from build123d import *

# Parameters (mm, degrees)
CROQUIS1_W              = 65
CROQUIS1_H              = 150
CROQUIS1_R              = 1.8
SALIENTE_EXTRUIR1_DEPTH = 2
CROQUIS2_W              = 3
CROQUIS2_H              = 150
SALIENTE_EXTRUIR2_DEPTH = 45
CROQUIS3_R              = 5.3
CROQUIS3_R_2            = 1.8
CORTAR_EXTRUIR1_DEPTH   = 10


with BuildPart() as part:
    # Croquis1 → Saliente-Extruir1 (new body)
    with BuildSketch(Plane(origin=(0, 0, 0), x_dir=(1, 0, 0), z_dir=(0, 1, 0))):
        Rectangle(CROQUIS1_W, CROQUIS1_H)
        with Locations(Location((-2.7, 12.25, 0), (0, 0, 270))):
            Circle(CROQUIS1_R, mode=Mode.SUBTRACT)
        with Locations(Location((-2.7, 60.57, 0), (0, 0, 270))):
            Circle(CROQUIS1_R, mode=Mode.SUBTRACT)
        with Locations(Location((-12.7, -60.57, 0), (0, 0, 90))):
            Circle(CROQUIS1_R, mode=Mode.SUBTRACT)
        with Locations(Location((-2.7, -60.57, 0), (0, 0, 90))):
            Circle(CROQUIS1_R, mode=Mode.SUBTRACT)
        with Locations(Location((-12.7, 12.25, 0), (0, 0, 270))):
            Circle(CROQUIS1_R, mode=Mode.SUBTRACT)
        with Locations(Location((-12.7, 60.57, 0), (0, 0, 270))):
            Circle(CROQUIS1_R, mode=Mode.SUBTRACT)
        with Locations(Location((-12.7, -12.25, 0), (0, 0, 90))):
            Circle(CROQUIS1_R, mode=Mode.SUBTRACT)
        with Locations(Location((-2.7, -12.25, 0), (0, 0, 90))):
            Circle(CROQUIS1_R, mode=Mode.SUBTRACT)
    extrude(amount=SALIENTE_EXTRUIR1_DEPTH)

    # Croquis2 → Saliente-Extruir2 (add)
    with BuildSketch(Plane(origin=(0, 2, 0), x_dir=(1, 0, 0), z_dir=(0, 1, 0))):
        with Locations((31, 0)):
            Rectangle(CROQUIS2_W, CROQUIS2_H)
    extrude(amount=SALIENTE_EXTRUIR2_DEPTH)

    # Croquis3 → Cortar-Extruir1 (cut)
    with BuildSketch(Plane(origin=(32.5, 0, 0), x_dir=(0, 0, -1), z_dir=(1, 0, 0))):
        with Locations((0, 23.5)):
            Circle(CROQUIS3_R)
        with Locations((-7.424621202, 16.075378798)):
            Circle(CROQUIS3_R_2)
        with Locations((-7.424621202, 30.924621202)):
            Circle(CROQUIS3_R_2)
        with Locations((7.424621202, 30.924621202)):
            Circle(CROQUIS3_R_2)
        with Locations((7.424621202, 16.075378798)):
            Circle(CROQUIS3_R_2)
    extrude(amount=-CORTAR_EXTRUIR1_DEPTH, mode=Mode.SUBTRACT)


solid = part.part
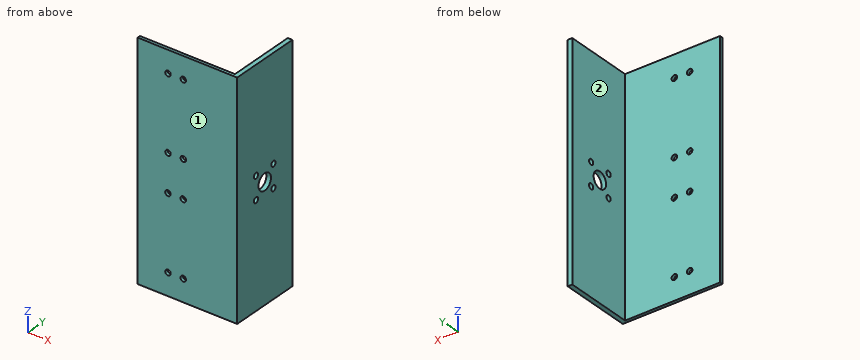
Build history of the part. All positions in model axes, mm. Face numbers are marked on the shaded views. A direction names the side the tool comes from. Coordinates: 2 decimals unless noted, no trailing zeros. Write each loop counter-clockwise with the first axis right and the second up, starting at its lowest first coordinate (ties: lowest second). Pieces come first, ordered by that corner, then holes.
(1) Pin check, flat tips, straight feed: pin 1 Ø17 at (y, z) = (23.5, 0) entering from +X; pin 2 Ø1 at (x, z) = (-18.5, 38.5) entering from +Y; pin 3 Ø8 at (y, z) = (36, -37) entering from -X. Stop position of each tip, or through.
(2) Cut at D-D on z = 41.5. List the corners of the cut face in (x, y), and give its area (3 significant figures).
(3) Cut at A-A on z = 0. List the corners of the cut face in (x, y), and give its area (3 significant figures).
(4) Cut at C-C on y = 23.5. List the corners of the cut face in (x, z).
(5) Drill centre lines: line 1 (X direction, y = 1, z = 12); line 2 (Y direction, x = 31.55, z = 0); line 3 (Y direction, x = 2, z = -32). Where is each one in solid material? Low to high.
(6) Cut at B-B on x = -2.7. List the corners of the cut face in (y, z).
(7) 3-axis set-ups, long thin cutter, end or side, ignore diameter. For the marked faces 1 and 2: which of +Z, -Z, +X, -X, +Y, -Y reach the whole face in a straight line?
Working result:
1. pin 1: stops at x = 32.5
1. pin 2: stops at y = 2
1. pin 3: stops at x = 29.5
2. outline: (-32.5, 0) - (32.5, 0) - (32.5, 47) - (29.5, 47) - (29.5, 2) - (-32.5, 2) - close
2. area: 265 mm2
3. outline: (-32.5, 0) - (32.5, 0) - (32.5, 18.2) - (29.5, 18.2) - (29.5, 2) - (-32.5, 2) - close; (29.5, 28.8) - (32.5, 28.8) - (32.5, 47) - (29.5, 47) - close
3. area: 233 mm2
4. outline: (29.5, -75) - (32.5, -75) - (32.5, -5.3) - (29.5, -5.3) - close; (29.5, 5.3) - (32.5, 5.3) - (32.5, 75) - (29.5, 75) - close
5. line 1: x = -32.5 to -14.48, -10.92 to -4.48, -0.92 to 32.5
5. line 2: y = 0 to 18.2, 28.8 to 47
5. line 3: y = 0 to 2
6. outline: (0, -75) - (2, -75) - (2, -62.37) - (0, -62.37) - close; (0, -58.77) - (2, -58.77) - (2, -14.05) - (0, -14.05) - close; (0, -10.45) - (2, -10.45) - (2, 10.45) - (0, 10.45) - close; (0, 14.05) - (2, 14.05) - (2, 58.77) - (0, 58.77) - close; (0, 62.37) - (2, 62.37) - (2, 75) - (0, 75) - close
7. face 1: +Z, -Z, +X, -X, -Y
7. face 2: +Z, -Z, -X, +Y
